```python
from build123d import *

# Parameters (mm, degrees)
F0_R     = 6.35
F1_DEPTH = 381
F2_R     = 12.7
F3_DEPTH = 12.7
F4_R     = 6.35
F5_DEPTH = 12.7


with BuildPart() as f1:
    # F0 (on Top) → F1 (new body)
    with BuildSketch(Plane.XY):
        Circle(F0_R)
    extrude(amount=-F1_DEPTH)

    # F2 (on Front) → F3 (join, symmetric)
    with BuildSketch(Plane.XZ):
        with Locations((0, 12.382501)):
            Circle(F2_R)
    extrude(amount=F3_DEPTH, both=True)

    # F4 (on Front) → F5 (cut, symmetric)
    with BuildSketch(Plane.XZ):
        with Locations((0, 12.110357)):
            Circle(F4_R)
    extrude(amount=F5_DEPTH, both=True, mode=Mode.SUBTRACT)


solid = f1.part
```
Source: CAD feature listing. Evaluate the final solid. Frame: model axes, mm. A direction names the side the tool comes from. Coordinates: 2 decimals unless noted, no trailing zeros. Loops run counter-clockwise (first coordinate to the right, second up) from the corner with the lowest first, then second, coordinate; pieces in that order, holes last. Notation, with made-up numbers: M 14,61.5 L 64,61.5 A15 cw 64,90.5 Z; hole C -24.5,13 d5. An arc over 180 degrees is marked long. Put each result on its own line as item: value. Start each with the question number.
1) Cut plane A-A on y = 0. Return the cut outline in (x, z), then the cut area to 3 significant figures.
2) Ray query, L1, parallel to Z at x = -0.5, y = -4.75; L2, parallel to Z at x = 0, y = 3.5; L3, parallel to Z at x = -4.5, y = 0.25. Return the intervals inside material, ascending. Write a range as from..to.
3) Pull-direction query (Z, two-part tool) for faces 1 (the face through (3, 12.7, 18)), 2 (the face through (0, 0, -381)), 3 (the face through (-0.827, -0.178, 18.406)); classes: pulls with the +Z half, pulls with the -Z half, needs draft (parallel to the pull), parting line crosses it, or undercut.
4) Reachability of faces 4 (the face through (3, -12.7, 18)), 5 (the face through (-1.38, -6.2, -187.83)) from +Z, -Z, +X, -X, +Y, -Y: full face, straight path, thin tool, end or side. Return the list, or none.
5) Cut plane B-B on z = -109.5. Return the cut outline in (x, y), then the cut area to 3 significant figures.
6) Contact query for flat-ended pins moving along their axis: pin 1 Ø3 at (x, y) = (-5.5, -2.5) entering from +Z; pin 2 Ø4 at (x, z) = (2.5, -130) entering from +Y; pin 3 Ø2 at (x, z) = (5, -296) entering from -Y. Output: stop coordinate, or through.
The answers:
1. outline: M -6.35,-381 L 6.35,-381 L 6.35,0 L 2.82,0 A12.7 ccw long -2.82,0 L -6.35,0 Z; hole C 0,12.11 d12.7
1. area: 5,220 mm²
2. L1: z = -381..5.78, 18.44..25.07
2. L2: z = -381..5.76, 18.46..25.08
2. L3: z = -381..0, 0.51..7.63, 16.59..24.26
3. face 1: needs draft
3. face 2: pulls with the -Z half
3. face 3: undercut
4. face 4: +Z, -Z, +X, -X, -Y
4. face 5: -Z
5. outline: C 0,0 d12.7
5. area: 127 mm²
6. pin 1: stops at z = 24.44
6. pin 2: stops at y = 6.33
6. pin 3: stops at y = -4.93
